For this review, take the finished solid that the model builds, in its own axes (mm). Face numbers are marked on the shaded views. Round coordinates to 2 decimals unless told otherwise and drop trailing zeros. Order: outer loops, then holes, each group sorted by start corner. A loop starts at its lowest first (then second) coordinate and runs counter-clockwise, first axis right, second up.
from build123d import *

# Parameters (mm, degrees)
SKETCH1_R               = 37.5
BOSS_EXTRUDE1_DEPTH     = 100
CUT_EXTRUDE1_DEPTH      = 114.192314227
CUT_EXTRUDE1_DEPTH_BACK = 114.192314227
SKETCH2_R               = 22.5
SKETCH3_W               = 11
SKETCH3_H               = 4
LPATTERN1_COUNT         = 19
LPATTERN1_PITCH         = 10


with BuildPart() as part:
    # Sketch1 → Boss-Extrude1 (new, symmetric)
    with BuildSketch(Plane(origin=(0, 0, 0), x_dir=(1, 0, 0), z_dir=(0, 1, 0))):
        with Locations(Location((0, 0, 0), (0, 0, 270))):
            Circle(SKETCH1_R)
    extrude(amount=BOSS_EXTRUDE1_DEPTH, both=True)

    # Sketch2 → Cut-Extrude1 (cut, two sides: drawn at the far end of the back side and taken through both)
    with BuildSketch(Plane(origin=(0, 0, 0), x_dir=(1, 0, 0), z_dir=(0, 1, 0)).offset(-CUT_EXTRUDE1_DEPTH_BACK)):
        with Locations(Location((0, 0, 0), (0, 0, 270))):
            Circle(SKETCH2_R)
    extrude(amount=CUT_EXTRUDE1_DEPTH + CUT_EXTRUDE1_DEPTH_BACK, mode=Mode.SUBTRACT)

    # Sketch3 → Cut-Revolve1 (revolve, cut)
    with BuildSketch(Plane.XY, mode=Mode.PRIVATE) as cut_revolve1_sk:
        with Locations((32, 90)):
            Rectangle(SKETCH3_W, SKETCH3_H)
    cut_revolve1 = revolve(cut_revolve1_sk.sketch.rotate(Axis((0, -110, 0), (0, 1, 0)), 90), axis=Axis((0, -110, 0), (0, 1, 0)), mode=Mode.SUBTRACT)

    # LPattern1: Cut-Revolve1 ×19
    with Locations(*[(0, -i * LPATTERN1_PITCH, 0) for i in range(1, LPATTERN1_COUNT)]):
        add(cut_revolve1, mode=Mode.SUBTRACT)


solid = part.part
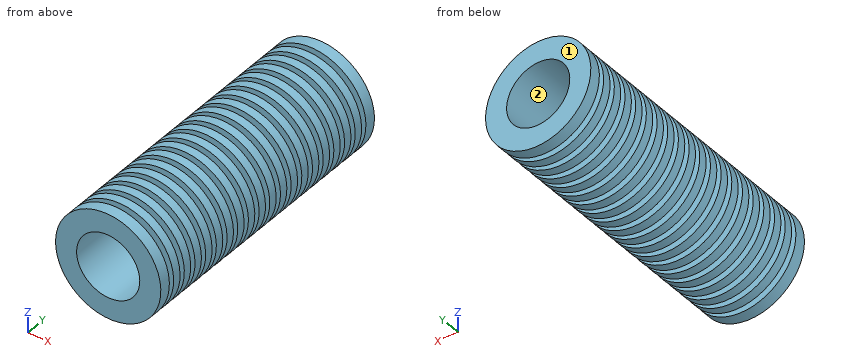
(1) Draft analysis for pull direction Z (two halves, no side actions). For the marked faces 1 and 2, state which applies: pulls with the +Z half, pulls with the -Z half, needs draft (parallel to the pull), parting line crosses it, or undercut.
(2) Clearance check with flat-ended pins moving along their axes: P1, Ø8, axis at x = 0.5, z = 15, coming from the -Y side; P2, Ø5, axis at y = 45.5, z = -5, coming from the -X side; P3, Ø10, axis at x = -6.5, y = 43, coming from the -Z side; P4, Ø5, axis at y = 71, z = -4, coming from the +X side. State where each tip first meets the part, or that it passes through.
(3) Add section B-B on x = 29. Count the separate pieces of the cut face and the enclosed holes in it, plus the area to 3 significant figures.
(4) Wall thickness on L1, parallel to X at y = -19, z = 0; L2, parallel to X at y = 33, z = 0: over which ranges is each line inside the solid? List them lowest first.
(5) Add section A-A on y = 40. Give the boundary of the cut face in (x, z), plus the area to 3 significant figures.
Here are the results:
1. face 1: needs draft
1. face 2: undercut
2. P1: passes through
2. P2: stops at x = -37.42
2. P3: stops at z = -37.47
2. P4: stops at x = 37.46
3. separate pieces: 20
3. enclosed holes: 0
3. area: 5,900 mm2
4. L1: x = -26.5 to -22.5, 22.5 to 26.5
4. L2: x = -37.5 to -22.5, 22.5 to 37.5
5. outline: circle Ø53 at (0, 0); hole circle Ø45 at (0, 0)
5. area: 616 mm2
